```python
from build123d import *

# Parameters (mm, degrees)
SKETCH_1_W          = 42.3
SKETCH_1_H          = 42.3
EXTRUDE_1_DEPTH     = 52
SKETCH_2_R          = 1.5
CUT_EXTRUDE_1_DEPTH = 4
SKETCH_3_R          = 11
EXTRUDE_2_DEPTH     = 2
SKETCH_4_R          = 2.5
EXTRUDE_3_DEPTH     = 20.5
CUT_EXTRUDE_START   = -18
CUT_EXTRUDE_4_DEPTH = 18
SKETCH_6_W          = 17
SKETCH_6_H          = 22
EXTRUDE_4_DEPTH     = 6


with BuildPart() as part:
    # 草图1 → 凸台-拉伸1 (new body)
    with BuildSketch(Plane(origin=(0, 0, 0), x_dir=(1, 0, 0), z_dir=(0, 1, 0))):
        Rectangle(SKETCH_1_W, SKETCH_1_H)
    extrude(amount=EXTRUDE_1_DEPTH)

    # 草图2 → 切除-拉伸1 (cut)
    with BuildSketch(Plane(origin=(0, 52, 0), x_dir=(1, 0, 0), z_dir=(0, 1, 0))):
        with Locations(Location((-15.5, 15.5, 0), (0, 0, 270))):
            Circle(SKETCH_2_R)
        with Locations(Location((15.5, 15.5, 0), (0, 0, 270))):
            Circle(SKETCH_2_R)
        with Locations(Location((15.5, -15.5, 0), (0, 0, 270))):
            Circle(SKETCH_2_R)
        with Locations(Location((-15.5, -15.5, 0), (0, 0, 270))):
            Circle(SKETCH_2_R)
    extrude(amount=-CUT_EXTRUDE_1_DEPTH, mode=Mode.SUBTRACT)

    # 草图3 → 凸台-拉伸2 (add)
    with BuildSketch(Plane(origin=(0, 52, 0), x_dir=(1, 0, 0), z_dir=(0, 1, 0))):
        with Locations(Location((0, 0, 0), (0, 0, 90))):
            Circle(SKETCH_3_R)
    extrude(amount=EXTRUDE_2_DEPTH)

    # 草图4 → 凸台-拉伸3 (add)
    with BuildSketch(Plane(origin=(0, 54, 0), x_dir=(1, 0, 0), z_dir=(0, 1, 0))):
        with Locations(Location((0, 0, 0), (0, 0, 270))):
            Circle(SKETCH_4_R)
    extrude(amount=EXTRUDE_3_DEPTH)

    # 草图5 → 切除-拉伸4 (cut)
    with BuildSketch(Plane(origin=(0, 74.5, 0), x_dir=(1, 0, 0), z_dir=(0, 1, 0)).offset(CUT_EXTRUDE_START)):
        with BuildLine():
            Line((2, 1.5), (2, -1.5))
            ThreePointArc((2, -1.5), (2.5, 0), (2, 1.5))
        make_face()
    extrude(amount=CUT_EXTRUDE_4_DEPTH, mode=Mode.SUBTRACT)

    # 草图6 → 凸台-拉伸4 (add)
    with BuildSketch(Plane.XY.offset(21.15)):
        with Locations((0, 11)):
            Rectangle(SKETCH_6_W, SKETCH_6_H)
    extrude(amount=EXTRUDE_4_DEPTH)


solid = part.part
```
Geometry check sheet. Reference: the model listing, model coordinates, mm. A direction names the side the tool comes from. Coordinates: 2 decimals unless noted, no trailing zeros. Loops run counter-clockwise (first coordinate to the right, second up) from the corner with the lowest first, then second, coordinate; pieces in that order, holes last. Notation, with made-up numbers: (48, 1) - (84, 1) arc R21 ccw to (84, 17) - close; hole circle Ø7 at (-31, 60.5). An arc over 180 degrees is marked (long way). One line per item, written item: value. Start each with the question number.
(1) Cross-section at D-D on z = 0. Enter the section's corners in (x, y), plus the area to 3 significant figures.
(2) Cross-section at B-B on x = -15.5. Enter the section's corners in (y, z).
(3) Depth check by flat-ended pin: P1, Ø3.5, axis at x = -15.5, z = -15.5, coming from the +Y side; P2, Ø0.9, axis at x = -15, z = -16, coming from the +Y side; P3, Ø3, axis at y = 10.5, z = 23, coming from the -X side. Enter the tip coordinate at first touch or a pass-through.
(4) Mould release check, pull along Z, two halves, no side actions. Record for faces 1 (the flat face through (-15, 48, 15)), 2 (the flat face through (16, 48, 15)), 3 (the flat face through (0, 74.5, 0)), 4 (the flat face through (0, 11, 27.15)): released by +Z, released by -Z, zero draft, split by the parting line, or undercut.
(5) Material ranges on line 1 (X direction, y = 49.25, z = 15.5); line 2 (Z direction, x = 15, y = 49); line 3 (Y direction, x = 16.5, z = -19), recorded low to high. Write a range as [from, to].
(6) Cross-section at A-A on z = -15.5. Enter the section's corners in (x, y).
(7) Cross-section at C-C on y = 13. Enter the section's corners in (x, z), plus the area to 3 significant figures.
(8) Tool access check on faces 5 (the flat face through (8.5, 11, 24)), 6 (the flat face through (-8.5, 11, 24)), 7 (the flat face through (-15, 48, -16)), 8 (the flat face through (0, 22, 24)). Record the directions out of +Z, -Z, +X, -X, +Y, -Y that give a thin tool (end or side, any length) a straight path to the whole face; none if there is none.
Results below:
1. outline: (-21.15, 0) - (21.15, 0) - (21.15, 52) - (11, 52) - (11, 54) - (2.5, 54) - (2.5, 56.5) - (2, 56.5) - (2, 74.5) - (-2.5, 74.5) - (-2.5, 54) - (-11, 54) - (-11, 52) - (-21.15, 52) - close
1. area: 2,340 mm2
2. outline: (0, -21.15) - (52, -21.15) - (52, -17) - (48, -17) - (48, -14) - (52, -14) - (52, 14) - (48, 14) - (48, 17) - (52, 17) - (52, 21.15) - (0, 21.15) - close
3. P1: stops at y = 52
3. P2: stops at y = 48
3. P3: stops at x = -8.5
4. face 1: undercut
4. face 2: undercut
4. face 3: zero draft
4. face 4: released by +Z
5. line 1: x = [-21.15, -17], [-14, 14], [17, 21.15]
5. line 2: z = [-21.15, -16.91], [-14.09, 14.09], [16.91, 21.15]
5. line 3: y = [0, 52]
6. outline: (-21.15, 0) - (21.15, 0) - (21.15, 52) - (17, 52) - (17, 48) - (14, 48) - (14, 52) - (-14, 52) - (-14, 48) - (-17, 48) - (-17, 52) - (-21.15, 52) - close
7. outline: (-21.15, -21.15) - (21.15, -21.15) - (21.15, 21.15) - (8.5, 21.15) - (8.5, 27.15) - (-8.5, 27.15) - (-8.5, 21.15) - (-21.15, 21.15) - close
7. area: 1,890 mm2
8. face 5: +Z, +X, +Y, -Y
8. face 6: +Z, -X, +Y, -Y
8. face 7: +Y
8. face 8: +Z, +X, -X, +Y
